```python
from build123d import *

# Parameters (mm, degrees)
SKETCH_R      = 100
SKETCH_R_2    = 20.3
PAD_DEPTH     = 10
SKETCH001_R   = 25
SKETCH001_R_2 = 20.3
PAD001_DEPTH  = 30


with BuildPart() as part:
    # Sketch → Pad (new body)
    with BuildSketch(Plane.XY):
        Circle(SKETCH_R)
        Circle(SKETCH_R_2, mode=Mode.SUBTRACT)
        with BuildLine():
            ThreePointArc((96.9497657449, 3.1213654066), (43.6438596811, 86.6268636864), (-55.1876984138, 79.7704076948))
            Line((-10.4473324135, 22.7124028989), (-55.1876984138, 79.7704076948))
            ThreePointArc((24.5596676208, 4.6714801032), (11.4524331511, 22.2225510443), (-10.4473324135, 22.7124028989))
            Line((24.5596676208, 4.6714801032), (96.9497657449, 3.1213654066))
        make_face(mode=Mode.SUBTRACT)
        with BuildLine():
            Line((24.7778278361, -3.3255447261), (96.9572766219, -2.8786298923))
            ThreePointArc((-51.0948365642, -82.4519112967), (45.9218644045, -85.441104684), (96.9572766219, -2.8786298923))
            Line((-11.1707596696, -22.3654673192), (-51.0948365642, -82.4519112967))
            ThreePointArc((-11.1707596696, -22.3654673192), (11.701185372, -22.0925838437), (24.7778278361, -3.3255447261))
        make_face(mode=Mode.SUBTRACT)
        with BuildLine():
            Line((-17.6635634383, -17.6917643739), (-56.0947674063, -79.1351822493))
            ThreePointArc((-60.0140125025, 76.2057629274), (-96.9691420251, -2.4465271145), (-56.0947674063, -79.1351822493))
            Line((-17.0867647821, 18.2494512049), (-60.0140125025, 76.2057629274))
            ThreePointArc((-17.0867647821, 18.2494512049), (-24.9967812363, 0.401158102), (-17.6635634383, -17.6917643739))
        make_face(mode=Mode.SUBTRACT)
    extrude(amount=PAD_DEPTH)

    # Sketch001 (on Face16 of Pad) → Pad001 (join)
    with BuildSketch(Plane.XY.offset(10)):
        Circle(SKETCH001_R)
        Circle(SKETCH001_R_2, mode=Mode.SUBTRACT)
    extrude(amount=PAD001_DEPTH)


solid = part.part
```
CAD build for the part. Positions are in the model's coordinates, mm. A direction names the side the tool comes from. Round coordinates to 2 decimals unless told otherwise and drop trailing zeros. Order: outer loops, then holes, each group sorted by start corner. A loop starts at its lowest first (then second) coordinate and runs counter-clockwise, first axis right, second up.
Item 1: Saw through at C-C on x = 76.5. Write the cut outline in (y, z).
Item 2: Tool access for faces 4 (the face through (44.94, 85.96, 4.93)), 5 (the face through (-15, 15, 0)): list every direction of +Z, -Z, +X, -X, +Y, -Y with a clear straight run to the whole face (end or side of a thin tool).
Item 3: Saw through at B-B on x = 0. Write the cut outline in (y, z), then the cut area to 3 significant figures.
Item 4: Saw through at D-D on z = 33. Write the cut outline in (x, y).
Item 5: Probe line 1 along Y through (x, z) = (0, 29.5); line 2 along X through (y, z) = (74.5, 7); line 3 along Y through (x, z) = (85, 3). List the from-to ranges inside material, lowest first.
Item 6: Mould opens along X. For faces 1 (the face through (95.38, 30.04, 4.93)), 2 (the face through (-15, 23, 10)), 3 (the face through (44.663, -86.106, 4.93)) say: pulls with the +X half, pulls with the -X half, needs draft (parallel to the pull), parting line crosses it, or undercut.
Item 7: Saw through at A-A on y = 0. Write the cut outline in (x, z), then the cut area to 3 significant figures.
Item 8: Pin check, flat tips, straight feed: pin 1 (6 mm diameter, centred on y = 39, z = 8, fed in from -X); pin 2 (6 mm diameter, centred on x = 60.5, z = 5.5, fed in from +Y); pin 3 (5 mm diameter, centred on y = -32.5, z = 9, fed in from -X). Stop position of each tip, or through.
Reported:
1. outline: (-64.4, 0) - (-59.64, 0) - (-59.64, 10) - (-64.4, 10) - close; (-3.01, 0) - (3.56, 0) - (3.56, 10) - (-3.01, 10) - close; (59.64, 0) - (64.4, 0) - (64.4, 10) - (59.64, 10) - close
2. face 4: +Z, -Z
2. face 5: -Z, +X, -X, +Y, -Y
3. outline: (-100, 0) - (-97, 0) - (-97, 10) - (-100, 10) - close; (-25, 0) - (-20.3, 0) - (-20.3, 40) - (-25, 40) - close; (20.3, 0) - (25, 0) - (25, 40) - (20.3, 40) - close; (97, 0) - (100, 0) - (100, 10) - (97, 10) - close
3. area: 436 mm2
4. outline: circle Ø50 at (0, 0); hole circle Ø40.6 at (0, 0)
5. line 1: y = -25 to -20.3, 20.3 to 25
5. line 2: x = -66.71 to -62.12, -58.75 to -51.06, 62.12 to 66.71
5. line 3: y = -52.68 to -46.73, -2.95 to 3.38, 46.73 to 52.68
6. face 1: parting line crosses it
6. face 2: needs draft
6. face 3: undercut
7. outline: (-100, 0) - (-97, 0) - (-97, 10) - (-100, 10) - close; (-25, 0) - (-20.3, 0) - (-20.3, 40) - (-25, 40) - close; (20.3, 0) - (100, 0) - (100, 10) - (25, 10) - (25, 40) - (20.3, 40) - close
7. area: 1,160 mm2
8. pin 1: stops at x = -93.3
8. pin 2: stops at y = 81.82
8. pin 3: stops at x = -95.39
